```python
from build123d import *

# Parameters (mm, degrees)
EXTRUDE_1_DEPTH = 3.75
SKETCH_4_R      = 0.75
SKETCH_4_R_2    = 0.5
EXTRUDE_3_DEPTH = 3.5
SKETCH_3_R      = 1.75
EXTRUDE_2_DEPTH = 2.45


with BuildPart() as part:
    # 草图2 → 凸台-拉伸1 (new body, symmetric)
    with BuildSketch(Plane(origin=(0, 0, 0), x_dir=(0, 0, -1), z_dir=(1, 0, 0))):
        Polygon((-2.55, 0), (4.45, 0), (4.45, 3), (3.45, 7), (-2.55, 7), align=None)
    extrude(amount=EXTRUDE_1_DEPTH, both=True)

    # 草图4 → 凸台-拉伸3 (add)
    with BuildSketch(Plane.XZ):
        with Locations((-3.5, -2.5)):
            Circle(SKETCH_4_R)
        with Locations((-2.25, 0)):
            Circle(SKETCH_4_R_2)
        with Locations((2.25, 0)):
            Circle(SKETCH_4_R_2)
        with Locations((3.5, -2.5)):
            Circle(SKETCH_4_R)
    extrude(amount=EXTRUDE_3_DEPTH)

    # 草图3 → 凸台-拉伸2 (add)
    with BuildSketch(Plane.XY.offset(2.55)):
        with Locations((0, 4)):
            Circle(SKETCH_3_R)
    extrude(amount=EXTRUDE_2_DEPTH)


solid = part.part
```
Geometry check sheet. Reference: the model listing, model coordinates, mm. A direction names the side the tool comes from. Coordinates: 2 decimals unless noted, no trailing zeros. Write each loop counter-clockwise with the first axis right and the second up, starting at its lowest first coordinate (ties: lowest second). Pieces come first, ordered by that corner, then holes. Notation, with made-up numbers: M -39.75,-12 L -4.75,-12 A19 cw -4.75,13 Z; hole C 28.5,87 d5. An arc over 180 degrees is marked long. One line per item, written item: value. Start each with the question number.
(1) Sectioned sample at B-B, the plane x = 2.25. Enter the section's corners in (y, z), and give its area (3 significant figures).
(2) Sectioned sample at D-D, the plane y = -1.25. Enter the section's corners in (x, z), and give its area (3 significant figures).
(3) Sectioned sample at C-C, the plane z = -2.5. Enter the section's corners in (x, y).
(4) Release check for a two-part mould opening along X. For faces 4 (the face through (0, 7, 0)), 5 (the face through (3.75, 4, -1)), 6 (the face through (-2.65, -1.73, -0.3)) record: released by +X, released by -X, zero draft, split by the parting line, or undercut.
(5) Scan lines: line 1 along X through (y, z) = (5.5, -0.75); line 2 along Z through (x, y) = (2.5, 1.5); line 3 along Y through (x, z) = (-1.5, -2). Record each from-to range of solid material in increasing order. Write a range as [from, to].
(6) Sectioned sample at A-A, the plane y = 4. Enter the section's corners in (x, z), and give its area (3 significant figures).
(7) Tool access check on faces 1 (the face through (3.5, -3.5, -2.5)), 2 (the face through (2.75, -1.73, -2.47)), 3 (the face through (-0.38, 2.29, 3.76)). Record the directions out of +Z, -Z, +X, -X, +Y, -Y that give a thin tool (end or side, any length) a straight path to the whole face; none if there is none.
(8) Depth check by flat-ended pin: pin 1 (1 mm diameter, centred on x = 0, z = 0.5, fed in from -Y); pin 2 (2 mm diameter, centred on y = 3.5, z = -2, fed in from -X). Enter the tip coordinate at first touch or a pass-through.
Filled sheet:
1. outline: M -3.5,-0.5 L 0,-0.5 L 0,-4.45 L 3,-4.45 L 7,-3.45 L 7,2.55 L 0,2.55 L 0,0.5 L -3.5,0.5 Z
1. area: 50.5 mm²
2. outline: C -3.5,-2.5 d1.5; C -2.25,0 d1; C 2.25,0 d1; C 3.5,-2.5 d1.5
2. area: 5.11 mm²
3. outline: M -4.25,-3.5 L -2.75,-3.5 L -2.75,0 L 2.75,0 L 2.75,-3.5 L 4.25,-3.5 L 4.25,0 L 3.75,0 L 3.75,7 L -3.75,7 L -3.75,0 L -4.25,0 Z
4. face 4: zero draft
4. face 5: released by +X
4. face 6: undercut
5. line 1: [-3.75, 3.75]
5. line 2: [-4.45, 2.55]
5. line 3: [0, 7]
6. outline: M -3.75,-4.2 L 3.75,-4.2 L 3.75,2.55 L 1.75,2.55 L 1.75,5 L -1.75,5 L -1.75,2.55 L -3.75,2.55 Z
6. area: 59.2 mm²
7. face 1: +Z, -Z, +X, -X, -Y
7. face 2: -Y
7. face 3: +Z
8. pin 1: y = 0
8. pin 2: x = -3.75
